Model file for the job. Use its own axes, mm. Face numbers are marked on the shaded views. A direction names the side the tool comes from. Round coordinates to 2 decimals unless told otherwise and drop trailing zeros. Loops run counter-clockwise (first coordinate to the right, second up) from the corner with the lowest first, then second, coordinate; pieces in that order, holes last. Notation, with made-up numbers: (56, -36) - (90, -36) arc R16 ccw to (90, -23) - close; hole circle Ø5 at (31.5, 37). An arc over 180 degrees is marked (long way). Use one line per item in the form item = value.
from build123d import *

# Parameters (mm, degrees)
FILLET1_R             = 0.2
SKETCH2_R             = 6.5
SKETCH2_R_2           = 4.6
CUT_EXTRUDE1_DEPTH    = 0.1
SKETCH3_W             = 2
SKETCH3_H             = 0.3
SKETCH3_W_2           = 0.3
SKETCH3_H_2           = 2
EXTRUDE_THIN1_DEPTH   = 7.6
CHAMFER1_SIZE         = 0.4
CHAMFER1_SIZE2        = 0.692820323
CHAMFER1_PART_2_SIZE  = 0.4
CHAMFER1_PART_2_SIZE2 = 0.692820323
CHAMFER1_PART_3_SIZE  = 0.4
CHAMFER1_PART_3_SIZE2 = 0.692820323
CHAMFER1_PART_4_SIZE  = 0.4
CHAMFER1_PART_4_SIZE2 = 0.692820323
CHAMFER2_SIZE         = 3
CHAMFER2_SIZE2        = 1.091910703


with BuildPart() as part:
    # Sketch1 → Revolve1 (revolve)
    with BuildSketch(Plane(origin=(0, 0, 0), x_dir=(0, 0, -1), z_dir=(1, 0, 0))):
        Polygon((0, 3.4), (-4.6, 3.4), (-4.6, 1.5), (-7, 1.5), (-9, 0.5), (-9, 0), (-8, 0), (-8, -18.6), (-5, -18.6), (-5, -26.4), (0, -26.4), align=None)
    revolve(axis=Axis((0, 14.375, 0), (0, -1, 0)))

    # Fillet1
    fillet1_edges = [part.edges().sort_by_distance(p)[0] for p in [
        (0, 3.4, -4.6),
    ]]
    fillet(fillet1_edges, radius=FILLET1_R)

    # Sketch2 → Cut-Extrude1 (cut)
    with BuildSketch(Plane(origin=(0, 1.5, 0), x_dir=(1, 0, 0), z_dir=(0, 1, 0))):
        Circle(SKETCH2_R)
        Circle(SKETCH2_R_2, mode=Mode.SUBTRACT)
    extrude(amount=-CUT_EXTRUDE1_DEPTH, mode=Mode.SUBTRACT)

    # Sketch3 → Extrude-Thin1 (add)
    with BuildSketch(Plane.XZ.offset(26.4)):
        with Locations((0, 4)):
            Rectangle(SKETCH3_W, SKETCH3_H)
        with Locations((0, -4)):
            Rectangle(SKETCH3_W, SKETCH3_H)
        with Locations((-4, 0)):
            Rectangle(SKETCH3_W_2, SKETCH3_H_2)
        with Locations((4, 1)):
            Rectangle(SKETCH3_W_2, SKETCH3_H_2)
    extrude(amount=EXTRUDE_THIN1_DEPTH)

    # Chamfer1
    chamfer1_edges = [part.edges().sort_by_distance(p)[0] for p in [
        (1, -34, 4),
        (-1, -34, 4),
    ]]
    chamfer1_side = [part.faces().sort_by_distance(p)[0] for p in [
        (0, -34, 4),
    ]]
    chamfer(chamfer1_edges, length=CHAMFER1_SIZE, length2=CHAMFER1_SIZE2, reference=chamfer1_side[0])

    # Chamfer1 part 2
    chamfer1_part_2_edges = [part.edges().sort_by_distance(p)[0] for p in [
        (1, -34, -4),
        (-1, -34, -4),
    ]]
    chamfer1_part_2_side = [part.faces().sort_by_distance(p)[0] for p in [
        (0, -34, -4),
    ]]
    chamfer(chamfer1_part_2_edges, length=CHAMFER1_PART_2_SIZE, length2=CHAMFER1_PART_2_SIZE2, reference=chamfer1_part_2_side[0])

    # Chamfer1 part 3
    chamfer1_part_3_edges = [part.edges().sort_by_distance(p)[0] for p in [
        (-4, -34, -1),
        (-4, -34, 1),
    ]]
    chamfer1_part_3_side = [part.faces().sort_by_distance(p)[0] for p in [
        (-4, -34, 0),
    ]]
    chamfer(chamfer1_part_3_edges, length=CHAMFER1_PART_3_SIZE, length2=CHAMFER1_PART_3_SIZE2, reference=chamfer1_part_3_side[0])

    # Chamfer1 part 4
    chamfer1_part_4_edges = [part.edges().sort_by_distance(p)[0] for p in [
        (4, -34, 2),
        (4, -34, 0),
    ]]
    chamfer1_part_4_side = [part.faces().sort_by_distance(p)[0] for p in [
        (4, -34, 1),
    ]]
    chamfer(chamfer1_part_4_edges, length=CHAMFER1_PART_4_SIZE, length2=CHAMFER1_PART_4_SIZE2, reference=chamfer1_part_4_side[0])

    # Chamfer2
    chamfer2_edges = [part.edges().sort_by_distance(p)[0] for p in [
        (0, -18.6, -8),
    ]]
    chamfer2_side = [part.faces().sort_by_distance(p)[0] for p in [
        (0, -9.3, -8),
    ]]
    chamfer(chamfer2_edges, length=CHAMFER2_SIZE, length2=CHAMFER2_SIZE2, reference=chamfer2_side[0])


solid = part.part
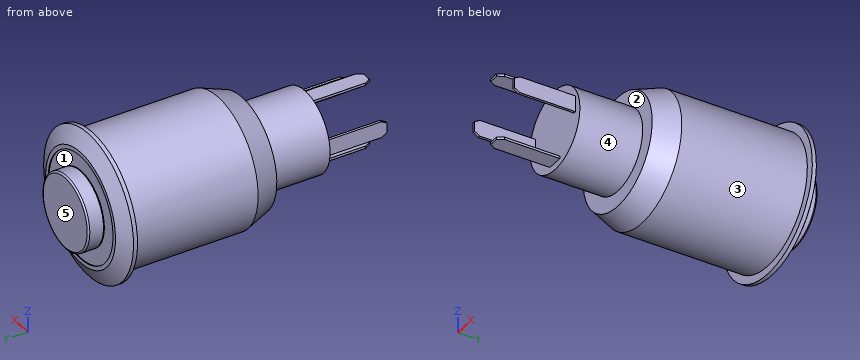
1. Cut at C-C, the plane y = -12. Give the cut face in (x, z).
Geometry check:
outline = circle Ø16 at (0, 0)
2. Tool access for the marked faces 4 and 5: list every direction of +Z, -Z, +X, -X, +Y, -Y with a clear straight run to the whole face (end or side of a thin tool).
Geometry check:
face_4 = -Y
face_5 = +Z, -Z, +X, -X, +Y
3. Wall check: probe 1 along Z at (x, y) = (0, 1.45); probe 2 along Y at (x, z) = (1.25, -0.5); probe 3 along X at (y, z) = (-31.5, -0.5). Give the ranges that are in metal, low to high.
Geometry check:
probe_1 = -7.1 to -6.5, -4.6 to 4.6, 6.5 to 7.1
probe_2 = -26.4 to 3.4
probe_3 = -4.15 to -3.85
4. Cut at A-A, the plane y = -28.5. Give the cut face in (x, z), plus the area to 3 significant figures.
Geometry check:
outline = (-4.15, -1) - (-3.85, -1) - (-3.85, 1) - (-4.15, 1) - close; (-1, -4.15) - (1, -4.15) - (1, -3.85) - (-1, -3.85) - close; (-1, 3.85) - (1, 3.85) - (1, 4.15) - (-1, 4.15) - close; (3.85, 0) - (4.15, 0) - (4.15, 2) - (3.85, 2) - close
area = 2.40 mm^2
5. Flat gauge pins, fed straight in: pin 1 (1.5 mm diameter, centred on y = -6, z = -2, fed in from +X); pin 2 (1.6 mm diameter, centred on y = -31, z = -0.5, fed in from -X); pin 3 (4 mm diameter, centred on x = -1, y = -14, fed in from -Z). Where does each tip first touch, or does it go through?
Geometry check:
pin_1 = 7.9
pin_2 = -4.15
pin_3 = -8
6. Pull direction Z, two halves, no side cores. Call the marked faces 1, 2 and 3: +Z half, -Z half, draft (parallel to the pull), parting line (faces both ways), or undercut.
Geometry check:
face_1 = undercut
face_2 = draft
face_3 = parting line
